Can you work these out from the model? Positions are in its coordinate system, mm. Face numbers are marked on the shaded views. A direction names the side the tool comes from. Coordinates: 2 decimals unless noted, no trailing zeros. Order: outer loops, then holes, each group sorted by start corner. A loop starts at its lowest first (then second) coordinate and runs counter-clockwise, first axis right, second up. Notation, with made-up numbers: (65.5, 84.5) -> (123.5, 84.5) arc R14 ccw to (123.5, 96.5) -> close; hole circle Ø10 at (26.25, 21.5). An arc over 180 degrees is marked (long way). Write item = value, one per line. Start each with the question number.
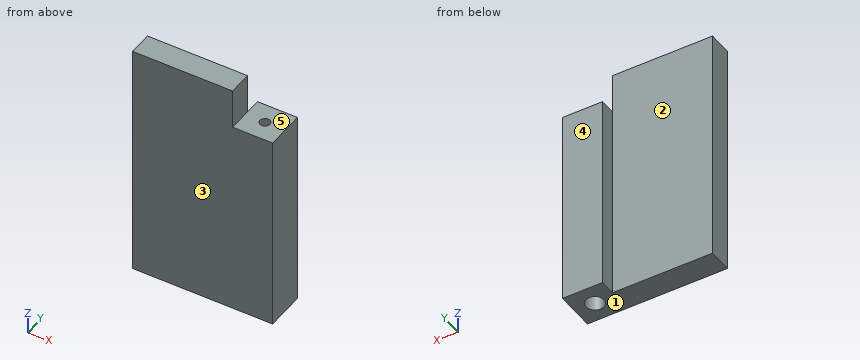
Autodesk Inventor part; units mm, degrees
ref_plane "YZ Plane" through (0, 0, 0) normal (1, 0, 0) x (0, 1, 0)
ref_plane "XZ Plane" through (0, 0, 0) normal (0, 1, 0) x (-1, 0, 0)
ref_plane "XY Plane" through (0, 0, 0) normal (0, 0, 1) x (1, 0, 0)
sketch "Sketch1" plane through (0, 0, 0) normal (0, 0, 1) x (1, 0, 0)
  line L0 (0, 20) -> (20, 20)
  line L1 (20, 20) -> (20, 0)
  line L2 (20, 0) -> (0, 0)
  line L3 (0, 0) -> (0, 20)
  circle A0 centre (10, 10) radius 2.5
  dimension "d0" = 20
  dimension "d1" = 20
  dimension "d5" = 10
  dimension "d6" = 10
  dimension "d7" = 5
extrude "Extrusion2" add sketch "Sketch1" along normal blind 25
sketch "Sketch4" plane through (0, 0, 25) normal (0, 0, 1) x (1, 0, 0)
  line L0 (0, 0) -> (20, 0)
  line L1 (0, 0) -> (-50, 0)
  line L2 (-50, 0) -> (-50, 12)
  line L3 (-50, 12) -> (0, 12)
  line L4 (0, 12) -> (0, 0)
  point P0 (0, 6)
  dimension "d13" = 12
  dimension "d14" = 50
extrude "Extrusion4" add sketch "Sketch4" against normal blind 100
sketch "Sketch5" plane through (0, 0, 0) normal (0, 0, -1) x (-1, 0, 0)
  line L0 (0, 0) -> (-20, 0)
  line L1 (-20, 0) -> (-20, 20)
  line L2 (0, 0) -> (-20, 0)
  line L3 (-20, 0) -> (-20, 20)
  line L4 (-20, 20) -> (0, 20)
  line L5 (0, 20) -> (0, 0)
  circle A0 centre (-10, 10) radius 2.5
  circle A1 centre (-10, 10) radius 4.5
  dimension "d17" = 9
extrude "Extrusion5" add sketch "Sketch5" along normal blind 75 contours L0 L1 L4 L5
sketch "Sketch6" plane through (0, 0, 25) normal (0, 0, 1) x (1, 0, 0)
  line L0 (-50, 0) -> (-50, 12)
  line L1 (0, 0) -> (-50, 0)
  line L2 (-50, 0) -> (-50, 12)
  line L3 (-50, 12) -> (0, 12)
  line L4 (0, 12) -> (0, 0)
extrude "Extrusion6" add sketch "Sketch6" along normal blind 20
properties part number "Touchscreen mount L v06"
(1) Thinking about a two-plate mould opening in Y: for the marked faces 3, 4 and 5, which applies, +Y half, -Y half, draft (parallel to the pull), parting line (faces both ways), or undercut?
(2) Imagine slicing it at C-C (x = 10). Write out the boundary of the cut face in (y, z), plus the area to 3 significant figures.
(3) Imagine slicing it at A-A (y = 10). Write out the boundary of the cut face in (x, z).
(4) Imagine slicing it at B-B (z = 20.5). Write out the boundary of the cut face in (x, y), plus the area to 3 significant figures.
(5) If I drill on L1, parallel to Y at x = 10, z = 10; L2, parallel to Y at x = 10, z = -39; L3, parallel to X at y = 9.5, z = -46.5, over which ranges is the centre line in solid material (lowest first)? Write a range as from..to.
(6) For the marked faces 1 and 2, which set-ups out of +Z, -Z, +X, -X, +Y, -Y let a thin tool reach every point of the face, with its end or its side?
(7) For P1, Ø2, axis at x = -35, z = 15.5, coming from the +Y side; P2, Ø2.5, axis at x = 8.5, y = 11, coming from the -Z side; P3, Ø3.5, axis at y = 4.5, z = 30, coming from the +X side, each with a flat end and sliding along its axis, tell me the tip position at first contact or that it passes through.
(8) Imagine slicing it at D-D (y = 2). Write out the boundary of the cut face in (x, z), plus the area to 3 significant figures.
Result set:
q1.face_3 = -Y half
q1.face_4 = +Y half
q1.face_5 = draft
q2.outline = (0, -75) -> (5.5, -75) -> (5.5, 0) -> (7.5, 0) -> (7.5, 25) -> (0, 25) -> close; (12.5, 0) -> (14.5, 0) -> (14.5, -75) -> (20, -75) -> (20, 25) -> (12.5, 25) -> close
q2.area = 1,200 mm2
q3.outline = (-50, -75) -> (5.5, -75) -> (5.5, 0) -> (7.5, 0) -> (7.5, 25) -> (0, 25) -> (0, 45) -> (-50, 45) -> close; (12.5, 0) -> (14.5, 0) -> (14.5, -75) -> (20, -75) -> (20, 25) -> (12.5, 25) -> close
q4.outline = (-50, 0) -> (20, 0) -> (20, 20) -> (0, 20) -> (0, 12) -> (-50, 12) -> close; hole circle Ø5 at (10, 10)
q4.area = 980 mm2
q5.L1 = 0..7.5, 12.5..20
q5.L2 = 0..5.5, 14.5..20
q5.L3 = -50..5.53, 14.47..20
q6.face_1 = -Z, +X, -X, +Y, -Y
q6.face_2 = +Z, -Z, -X, +Y
q7.P1 = 12
q7.P2 = 0
q7.P3 = 0
q8.outline = (-50, -75) -> (20, -75) -> (20, 25) -> (0, 25) -> (0, 45) -> (-50, 45) -> close
q8.area = 8,000 mm2
